Design review of the part built by this model. Coordinates are the model's own, in mm. Face numbers are marked on the shaded views. A direction names the side the tool comes from. Give positions to 0.01 mm unless a question says otherwise; leave off trailing zeros. Order: outer loops, then holes, each group sorted by start corner. A loop starts at its lowest first (then second) coordinate and runs counter-clockwise, first axis right, second up. Notation, with made-up numbers: M 33.25,62.5 L 65.25,62.5 A28 ccw 65.25,88.5 Z; hole C 10.25,67.25 d10. An arc over 180 degrees is marked long. Answer as a JSON object with one key per item and string values.
from build123d import *

# Parameters (mm, degrees)
SKETCH2_R               = 2.38125
CUT_EXTRUDE1_DEPTH      = 1
CUT_EXTRUDE1_DEPTH_BACK = 10.525
CHAMFER1_SIZE           = 0.396875


with BuildPart() as part:
    # Sketch1 → Revolve1 (revolve)
    with BuildSketch(Plane.XY):
        Polygon((0, 0), (9.525, 0), (9.525, 0.79375), (6.35, 2.38125), (6.35, 7.14375), (9.525, 8.73125), (9.525, 9.525), (0, 9.525), align=None)
    revolve(axis=Axis((0, 9.525, 0), (0, -1, 0)))

    # Sketch2 → Cut-Extrude1 (cut, two sides)
    with BuildSketch(Plane(origin=(0, 9.525, 0), x_dir=(1, 0, 0), z_dir=(0, 1, 0))) as cut_extrude1_sk:
        Circle(SKETCH2_R)
    extrude(amount=CUT_EXTRUDE1_DEPTH, mode=Mode.SUBTRACT)
    extrude(cut_extrude1_sk.sketch, amount=-CUT_EXTRUDE1_DEPTH_BACK, mode=Mode.SUBTRACT)

    # Chamfer1
    chamfer1_edges = [part.edges().sort_by_distance(p)[0] for p in [
        (-2.38125, 0, 0),
        (-2.38125, 9.525, 0),
        (-9.525, 9.525, 0),
        (-9.525, 0, 0),
    ]]
    chamfer(chamfer1_edges, length=CHAMFER1_SIZE)


solid = part.part
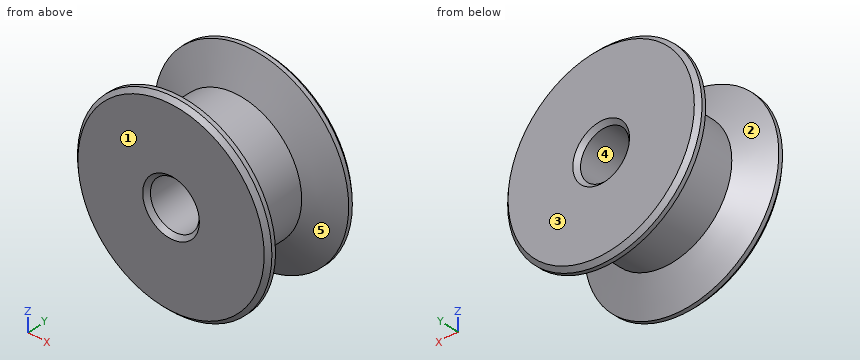
(1) We need section B-B (x = 0). Write out the cut boundary in (y, z) (3 decimals), plus the area to 3 significant figures.
Checked values:
{"outline": "M 0,-9.128 L 0.397,-9.525 L 0.794,-9.525 L 2.381,-6.35 L 7.144,-6.35 L 8.731,-9.525 L 9.128,-9.525 L 9.525,-9.128 L 9.525,-2.778 L 9.128,-2.381 L 0.397,-2.381 L 0,-2.778 Z; M 0,2.778 L 0.397,2.381 L 9.128,2.381 L 9.525,2.778 L 9.525,9.128 L 9.128,9.525 L 8.731,9.525 L 7.144,6.35 L 2.381,6.35 L 0.794,9.525 L 0.397,9.525 L 0,9.128 Z", "area": "95.1 mm^2"}
(2) Insertion check: pin 1 (5 mm diameter, centred on x = 4.5, y = 4.5, fed in from -Z). The pin has a flat end and moves straight along its axis. Give the tip position at first contact, or say it passes through.
Checked values:
{"pin 1": "stops at z = -6.03"}
(3) We need section A-A (z = 0). Write out the cut boundary in (x, y) (3 decimals), plus the area to 3 significant figures.
Checked values:
{"outline": "M -9.525,0.397 L -9.128,0 L -2.778,0 L -2.381,0.397 L -2.381,9.128 L -2.778,9.525 L -9.128,9.525 L -9.525,9.128 L -9.525,8.731 L -6.35,7.144 L -6.35,2.381 L -9.525,0.794 Z; M 2.381,0.397 L 2.778,0 L 9.128,0 L 9.525,0.397 L 9.525,0.794 L 6.35,2.381 L 6.35,7.144 L 9.525,8.731 L 9.525,9.128 L 9.128,9.525 L 2.778,9.525 L 2.381,9.128 Z", "area": "95.1 mm^2"}
(4) We need section D-D (y = 8.25). Write out the cut boundary in (x, z) (1 decimal).
Checked values:
{"outline": "C 0,0 d17.1; hole C 0,0 d4.8"}
(5) To check wall thickness, follow L1, parallel to Z at x = 0, y = 4.25; L2, parallel to X at y = 2.25, z = -1.25; L3, parallel to Y at x = -3.75, z = -8.5. State the ranges of each line that lie inside material, in increasing order. Write a range as from..to.
Checked values:
{"L1": "z = -6.35..-2.38, 2.38..6.35", "L2": "x = -6.49..-2.03, 2.03..6.49", "L3": "y = 0.16..0.91, 8.61..9.36"}
(6) Tool access review of the marked faces 1 and 2: name each direction out of +Z, -Z, +X, -X, +Y, -Y from which nothing blocks a thin tool from reaching the whole face with its end or side.
Checked values:
{"face 1": "+Z, -Z, +X, -X, -Y", "face 2": "none"}
(7) We need section C-C (y = 3.75). Write out the cut boundary in (x, z).
Checked values:
{"outline": "C 0,0 d12.7; hole C 0,0 d4.76"}
(8) Draft analysis for pull direction X (two halves, no side actions). For the marked faces 3, 4 and 5, state which applies: +X half, -X half, draft (parallel to the pull), parting line (faces both ways), or undercut.
Checked values:
{"face 3": "draft", "face 4": "undercut", "face 5": "parting line"}
